Here's how the part is built. I have some questions about the finished solid (model axes, mm). A direction names the side the tool comes from. Give positions to 0.01 mm unless a question says otherwise; leave off trailing zeros. Order: outer loops, then holes, each group sorted by start corner. A loop starts at its lowest first (then second) coordinate and runs counter-clockwise, first axis right, second up. Notation, with made-up numbers: M -30.75,75 L -11.75,75 A30 ccw -11.75,113 Z; hole C 75.25,58 d11. An arc over 180 degrees is marked long. Use one line per item in the form item = value.
from build123d import *

# Parameters (mm, degrees)
SKETCH1_W           = 20
SKETCH1_H           = 30
BOSS_EXTRUDE1_DEPTH = 60
SKETCH2_W           = 20
SKETCH2_H           = 50
SKETCH2_R           = 2.25
BOSS_EXTRUDE2_DEPTH = 4
CUT_EXTRUDE1_DEPTH  = 41
FILLET1_R           = 4
SKETCH4_W           = 10
SKETCH4_H           = 20
CUT_EXTRUDE2_DEPTH  = 5
CHAMFER1_SIZE       = 14
CHAMFER1_SIZE2      = 16.684550296


with BuildPart() as part:
    # Sketch1 → Boss-Extrude1 (new body)
    with BuildSketch(Plane(origin=(0, 0, 0), x_dir=(0, 0, -1), z_dir=(1, 0, 0))):
        with Locations((10, 15)):
            Rectangle(SKETCH1_W, SKETCH1_H)
    extrude(amount=BOSS_EXTRUDE1_DEPTH)

    # Sketch2 → Boss-Extrude2 (add)
    with BuildSketch(Plane(origin=(0, 0, -20), x_dir=(-1, 0, 0), z_dir=(0, 0, -1))):
        with Locations((-10, 15)):
            Rectangle(SKETCH2_W, SKETCH2_H)
        with Locations((-10, 35)):
            Circle(SKETCH2_R, mode=Mode.SUBTRACT)
        with Locations((-10, -5)):
            Circle(SKETCH2_R, mode=Mode.SUBTRACT)
    extrude(amount=-BOSS_EXTRUDE2_DEPTH)

    # Sketch3 → Cut-Extrude1 (cut, through all)
    with BuildSketch(Plane(origin=(0, 30, 0), x_dir=(1, 0, 0), z_dir=(0, 1, 0))):
        Polygon((60, 20), (40, 20), (60, 0), align=None)
    extrude(amount=-CUT_EXTRUDE1_DEPTH, mode=Mode.SUBTRACT)

    # Fillet1
    fillet1_edges = [part.edges().sort_by_distance(p)[0] for p in [
        (60, 15, 0),
    ]]
    fillet(fillet1_edges, radius=FILLET1_R)

    # Sketch4 → Cut-Extrude2 (cut)
    with BuildSketch(Plane(origin=(30, 0, -30), x_dir=(-0.707106781, 0, -0.707106781), z_dir=(0.707106781, 0, -0.707106781))):
        with Locations((-26.142135624, 15)):
            Rectangle(SKETCH4_W, SKETCH4_H)
    extrude(amount=-CUT_EXTRUDE2_DEPTH, mode=Mode.SUBTRACT)

    # Chamfer1
    chamfer1_edges = [part.edges().sort_by_distance(p)[0] for p in [
        (0, 15, 0),
    ]]
    chamfer1_side = [part.faces().sort_by_distance(p)[0] for p in [
        (0, 15, -10.941176471),
    ]]
    chamfer(chamfer1_edges, length=CHAMFER1_SIZE, length2=CHAMFER1_SIZE2, reference=chamfer1_side[0])


solid = part.part
Q1. I want a section at C-C on y = 9. Write out the boundary of the cut face in (x, z), then the cut area to 3 significant figures.
Found:
outline = M 0,-20 L 40,-20 L 44.95,-15.05 L 41.41,-11.51 L 48.49,-4.44 L 52.02,-7.98 L 53.17,-6.83 A4 ccw 50.34,0 L 16.68,0 L 0,-14 Z
area = 813 mm²
Q2. Thinking about a two-plate mould opening in Y: for faces 5 (the face through (10, 40, -18)), 6 (the face through (12.4, -4.9, -16)), 7 (the face through (12.248, -4.901, -18.028)), which applies, +Y half, -Y half, draft (parallel to the pull), parting line (faces both ways), or undercut?
Found:
face_5 = +Y half
face_6 = draft
face_7 = undercut
Q3. I'm going to push flat-ended pins straight in: pin 1 Ø6 at (y, z) = (4, -4) entering from -X; pin 2 Ø3 at (y, z) = (-6.5, -17.5) entering from +X; pin 3 Ø6 at (x, z) = (34, -10) entering from +Y. Where does each tip first touch, or does it pass through?
Found:
pin_1 = 8.34
pin_2 = 20
pin_3 = 30
Q4. I want a section at B-B on x = 10. Write out the boundary of the cut face in (y, z), then the cut area to 3 significant figures.
Found:
outline = M -10,-20 L -7.25,-20 L -7.25,-16 L -10,-16 Z; M -2.75,-20 L 32.75,-20 L 32.75,-16 L 30,-16 L 30,-5.61 L 0,-5.61 L 0,-16 L -2.75,-16 Z; M 37.25,-20 L 40,-20 L 40,-16 L 37.25,-16 Z
area = 476 mm²
Q5. I need wall thicknesses on L1, parallel to Y at x = 10, z = -18.4; L2, parallel to Z at x = 7.5, y = 37.5; L3, parallel to Y at x = 39.5, z = -10.5. Which ranges of each line are inside material? Lowest first, please.
Found:
L1 = -10 to -7.25, -2.75 to 32.75, 37.25 to 40
L2 = -20 to -16
L3 = 0 to 30
Q6. On a 3-axis mill with a long thin cutter (end or side, diameter ignored), from which of +Z, -Z, +X, -X, +Y, -Y can I reach the whole of each face in a straight line? I mean faces 1 (the face through (43.2, 14.9, -13.3)), 2 (the face through (20, -5, -18)), 3 (the face through (20, 35, -18)), 4 (the face through (47, 5, -10)). Say none if no direction works.
Found:
face_1 = +X
face_2 = +Z, -Z, +X, -Y
face_3 = +Z, -Z, +X, +Y
face_4 = none
Q7. I want a section at A-A on y = -5. Write out the boundary of the cut face in (x, z), then the cut area to 3 significant figures.
Found:
outline = M 0,-20 L 7.75,-20 L 7.75,-16 L 0,-16 Z; M 12.25,-20 L 20,-20 L 20,-16 L 12.25,-16 Z
area = 62.0 mm²
Q8. I want a section at D-D on z = -13. Write out the boundary of the cut face in (x, y), then the cut area to 3 significant figures.
Found:
outline = M 1.19,0 L 47,0 L 47,5 L 42.9,5 L 42.9,25 L 47,25 L 47,30 L 1.19,30 Z
area = 1,290 mm²
